Source: CAD feature listing. Evaluate the final solid. Frame: model axes, mm. A direction names the side the tool comes from. Give positions to 0.01 mm unless a question says otherwise; leave off trailing zeros. Write each loop counter-clockwise with the first axis right and the second up, starting at its lowest first coordinate (ties: lowest second). Pieces come first, ordered by that corner, then holes. Notation, with made-up numbers: (62, 71.5) -> (104, 71.5) arc R29 ccw to (104, 107.5) -> close; hole circle Ø4 at (-25.75, -30.5). An arc over 180 degrees is marked (long way). Write item = value, one per line.
from build123d import *

# Parameters (mm, degrees)
SKETCH2_W               = 14.5
SKETCH2_H               = 15
OUTLINE_EXTRUSION_DEPTH = 12.7
SKETCH3_W               = 12
SKETCH3_H               = 7.2
SKETCH3_W_2             = 4
SKETCH3_H_2             = 1.06471969
SKETCH3_W_3             = 0.9
SKETCH3_H_3             = 2.5
CUT_EXTRUDE1_DEPTH      = 14
SKETCH5_R               = 0.45
CUT_EXTRUDE2_DEPTH      = 14
SKETCH6_W               = 4
SKETCH6_H               = 0.1
BOSS_EXTRUDE1_DEPTH     = 11.5
SKETCH7_W               = 1.2
SKETCH7_H               = 0.96471969
CUT_EXTRUDE3_DEPTH      = 13


with BuildPart() as part:
    # Sketch2 → Outline extrusion (new body)
    with BuildSketch(Plane(origin=(0, 0, 0), x_dir=(1, 0, 0), z_dir=(0, 1, 0))):
        Rectangle(SKETCH2_W, SKETCH2_H)
    extrude(amount=OUTLINE_EXTRUSION_DEPTH)

    # Sketch3 → Cut-Extrude1 (cut)
    with BuildSketch(Plane.XY.offset(7.5)):
        with Locations((0, 5.795210166)):
            Rectangle(SKETCH3_W, SKETCH3_H)
        Polygon((-3.2, 11.030490476), (-3.2, 9.395210166), (3.2, 9.395210166), (3.2, 11.030490476), (2, 11.030490476), (-2, 11.030490476), align=None)
        with Locations((0, 11.562850321)):
            Rectangle(SKETCH3_W_2, SKETCH3_H_2)
        with Locations((6.45, 6.883168125)):
            Rectangle(SKETCH3_W_3, SKETCH3_H_3)
        with Locations((-6.45, 6.883168125)):
            Rectangle(SKETCH3_W_3, SKETCH3_H_3)
    extrude(amount=-CUT_EXTRUDE1_DEPTH, mode=Mode.SUBTRACT)

    # Sketch5 → Cut-Extrude2 (cut)
    with BuildSketch(Plane.XY.offset(7.5)):
        with Locations((-6, 11.030490476)):
            Circle(SKETCH5_R)
    extrude(amount=-CUT_EXTRUDE2_DEPTH, mode=Mode.SUBTRACT)

    # Sketch6 → Boss-Extrude1 (add)
    with BuildSketch(Plane.XY.offset(-6.5)):
        with Locations((0, 12.045210166)):
            Rectangle(SKETCH6_W, SKETCH6_H)
    extrude(amount=BOSS_EXTRUDE1_DEPTH)

    # Sketch7 → Cut-Extrude3 (cut)
    with BuildSketch(Plane.XY.offset(-6.5)):
        with Locations((-2.6, 11.512850321)):
            Rectangle(SKETCH7_W, SKETCH7_H)
        with Locations((2.6, 11.512850321)):
            Rectangle(SKETCH7_W, SKETCH7_H)
    extrude(amount=CUT_EXTRUDE3_DEPTH, mode=Mode.SUBTRACT)


solid = part.part
(1) Access query for faces 4 (the face through (0, 12.7, 0)), 5 (the face through (-6.9, 7, 1)), 6 (the face through (-3.2, 11, 0)). Directions: +Z, -Z, +X, -X, +Y, -Y. A direction counts if a zero-diameter tool reaches every point of the face in a straight line with its end or side. Return the directions, or none.
Values follow:
face_4 = +Z, -Z, +X, -X, +Y
face_5 = +Z
face_6 = none
(2) Pull-direction query (Z, two-part tool) for faces 1 (the face through (0, 6, -7.5)), 2 (the face through (7.25, 6, 0)), 3 (the face through (2.6, 11.5, 6.5)); classes: pulls with the +Z half, pulls with the -Z half, needs draft (parallel to the pull), parting line crosses it, or undercut.
Values follow:
face_1 = pulls with the -Z half
face_2 = needs draft
face_3 = undercut
(3) Section query A-A (y = 3.5). Return loops of the section in (x, z).
Values follow:
outline = (-7.25, -7.5) -> (7.25, -7.5) -> (7.25, 7.5) -> (6, 7.5) -> (6, -6.5) -> (-6, -6.5) -> (-6, 7.5) -> (-7.25, 7.5) -> close
(4) Section query C-C (x = 3.5). Return loops of the section in (y, z), plus the area to 3 significant figures.
Values follow:
outline = (0, -7.5) -> (12.7, -7.5) -> (12.7, 7.5) -> (9.4, 7.5) -> (9.4, -6.5) -> (2.2, -6.5) -> (2.2, 7.5) -> (0, 7.5) -> close
area = 89.7 mm2
(5) Section query B-B (z = 0.5). Return loops of the section in (x, y).
Values follow:
outline = (-7.25, 0) -> (7.25, 0) -> (7.25, 12.7) -> (-7.25, 12.7) -> close; hole (-6.9, 5.63) -> (-6, 5.63) -> (-6, 2.2) -> (6, 2.2) -> (6, 5.63) -> (6.9, 5.63) -> (6.9, 8.13) -> (6, 8.13) -> (6, 9.4) -> (3.2, 9.4) -> (3.2, 12) -> (-3.2, 12) -> (-3.2, 9.4) -> (-6, 9.4) -> (-6, 8.13) -> (-6.9, 8.13) -> close; hole circle Ø0.9 at (-6, 11.03)
(6) Section query D-D (y = 11.25). Return loops of the section in (x, z).
Values follow:
outline = (-7.25, -7.5) -> (7.25, -7.5) -> (7.25, 7.5) -> (2, 7.5) -> (2, 6.5) -> (3.2, 6.5) -> (3.2, -6.5) -> (-3.2, -6.5) -> (-3.2, 6.5) -> (-2, 6.5) -> (-2, 7.5) -> (-5.61, 7.5) -> (-5.61, -6.5) -> (-6.39, -6.5) -> (-6.39, 7.5) -> (-7.25, 7.5) -> close
(7) Material intervals for line 1 (X direction, y = 7.25, z = 6.25); line 2 (X direction, y = 9.25, z = 6.75); line 3 (Y direction, x = 3.25, z = 1.75), sorted ascending.
Values follow:
line_1 = -7.25 to -6.9, 6.9 to 7.25
line_2 = -7.25 to -6, 6 to 7.25
line_3 = 0 to 2.2, 9.4 to 12.7
(8) First-contact query: pin 1 (3 mm diameter, centred on x = 2.5, y = 6.5, fed in from +Z). Flat tip, straight axial feed; report the tip coordinate or a pass-through.
Values follow:
pin_1 = -6.5
